from build123d import *

# Parameters (mm, degrees)
BOSS_EXTRUDE1_DEPTH = 30.48
BOSS_EXTRUDE2_DEPTH = 3.175
SKETCH3_W           = 3.436
SKETCH3_H           = 3.81
CUT_EXTRUDE1_DEPTH  = 12.7
SKETCH5_R           = 2.45
CUT_EXTRUDE2_DEPTH  = 1.5875
SKETCH6_W           = 23
SKETCH6_H           = 27.305
SKETCH6_R           = 4.5
BOSS_EXTRUDE3_DEPTH = 3.2
FILLET3_R           = 0.5
FILLET1_R           = 0.5
FILLET5_R           = 0.5
FILLET4_R           = 0.5
FILLET6_R           = 0.5


with BuildPart() as part:
    # Sketch1 → Boss-Extrude1 (new body)
    with BuildSketch(Plane(origin=(0, 0, 0), x_dir=(1, 0, 0), z_dir=(0, 1, 0))):
        Polygon((4.5, -6.1), (4.5, -7.6875), (13.088, -7.6875), (13.088, 7.6875), (-13.088, 7.6875), (-13.088, -7.6875), (-4.5, -7.6875), (-4.5, -6.1), (-11.5, -6.1), (-11.5, 6.1), (11.5, 6.1), (11.5, -6.1), align=None)
    extrude(amount=BOSS_EXTRUDE1_DEPTH)

    # Sketch2 → Boss-Extrude2 (add)
    with BuildSketch(Plane.XZ):
        Polygon((11.5, 0), (11.5, 6.1), (9.5, 6.1), (9.5, 0), (-1.5, 0), (-1.5, 6.1), (-11.5, 6.1), (-11.5, -6.1), (11.5, -6.1), align=None)
    extrude(amount=-BOSS_EXTRUDE2_DEPTH)

    # Sketch3 → Cut-Extrude1 (cut)
    with BuildSketch(Plane(origin=(0, 30.48, 0), x_dir=(1, 0, 0), z_dir=(0, 1, 0))):
        with Locations((-11.37, -2.925)):
            Rectangle(SKETCH3_W, SKETCH3_H)
    cut_extrude1 = extrude(amount=-CUT_EXTRUDE1_DEPTH, mode=Mode.SUBTRACT)

    # Mirror1: Cut-Extrude1 across plane
    add(cut_extrude1.mirror(Plane(origin=(0, 0, 0), x_dir=(0, 0, 1), z_dir=(1, 0, 0))), mode=Mode.SUBTRACT)

    # Sketch5 → Cut-Extrude2 (cut)
    with BuildSketch(Plane(origin=(0, 0, -7.6875), x_dir=(-1, 0, 0), z_dir=(0, 0, -1))):
        with Locations((0, 8.466666667)):
            Circle(SKETCH5_R)
        with Locations((0, 22.013333333)):
            Circle(SKETCH5_R)
    extrude(amount=-CUT_EXTRUDE2_DEPTH, mode=Mode.SUBTRACT)

    # Sketch6 → Boss-Extrude3 (add)
    with BuildSketch(Plane.XY.offset(-6.1)):
        with Locations((0, 16.8275)):
            Rectangle(SKETCH6_W, SKETCH6_H)
        with Locations((0, 22.013333333)):
            Circle(SKETCH6_R, mode=Mode.SUBTRACT)
        with Locations((0, 8.466666667)):
            Circle(SKETCH6_R, mode=Mode.SUBTRACT)
    extrude(amount=BOSS_EXTRUDE3_DEPTH)

    # Fillet3
    fillet3_edges = [part.edges().sort_by_distance(p)[0] for p in [
        (11.5, 3.175, 1.6),
        (0, 3.175, -2.9),
        (11.5, 16.8275, -2.9),
        (11.5, 16.8275, 6.1),
    ]]
    fillet(fillet3_edges, radius=FILLET3_R)

    # Fillet1
    fillet1_edges = [part.edges().sort_by_distance(p)[0] for p in [
        (-11.5, 17.0775, -2.9),
        (-11.5, 3.321446609, -2.753553391),
        (4.5, 15.24, 6.1),
        (-11.5, 3.175, 1.85),
        (-8, 3.175, 6.1),
    ]]
    fillet(fillet1_edges, radius=FILLET1_R)

    # Fillet5
    # the kernel refuses this fillet: 0.5 mm, written as the material it adds along each edge
    with BuildSketch(Plane(origin=(-13.088, 17.78, 4.83), x_dir=(0, 1, 0), z_dir=(1, 0, 0)), Plane(origin=(11.5, 17.78, 1.02), x_dir=(0, 0, 1), z_dir=(1, 0, 0))) as fillet5_piece_1:
        with BuildLine():
            CenterArc((FILLET5_R, -FILLET5_R), FILLET5_R, 90, 90)
            Line((0, -FILLET5_R), (0, 0))
            Line((0, 0), (FILLET5_R, 0))
        make_face()
    extrude(amount=1.588)
    with BuildSketch(Plane(origin=(-11.5, 17.78, 1.02), x_dir=(0, 0, 1), z_dir=(-1, 0, 0)), Plane(origin=(13.088, 17.78, 4.83), x_dir=(0, 1, 0), z_dir=(-1, 0, 0))) as fillet5_piece_2:
        with BuildLine():
            CenterArc((FILLET5_R, FILLET5_R), FILLET5_R, 180, 90)
            Line((0, FILLET5_R), (0, 0))
            Line((0, 0), (FILLET5_R, 0))
        make_face()
    extrude(amount=1.588)
    # the kernel refuses this fillet: 0.5 mm, written as the material it takes off along each edge
    with BuildSketch(Plane(origin=(-4.5, 3.675, 6.1), x_dir=(0, 0, 1), z_dir=(0, 1, 0))) as fillet5_2_piece_1:
        with BuildLine():
            CenterArc((FILLET5_R, -FILLET5_R), FILLET5_R, 90, 90)
            Line((0, -FILLET5_R), (0, 0))
            Line((0, 0), (FILLET5_R, 0))
        make_face()
    extrude(amount=28.055, mode=Mode.SUBTRACT)
    with BuildSketch(Plane(origin=(-4.5, 3.675, 5.6), x_dir=(0, 0.8017442392976493, -0.5976672776328263), z_dir=(0, 0.5976672776328263, 0.8017442392976493))) as fillet5_2_piece_2_section:
        with BuildLine():
            CenterArc((0.5 + FILLET5_R, FILLET5_R), FILLET5_R, 180, 90)
            Line((0.5, FILLET5_R), (0.5, 0))
            Line((0.5, 0), (0.5 + FILLET5_R, 0))
        make_face()
    fillet5_2_piece_2 = revolve(axis=Axis((-4.5, 3.675, 5.6), (-1, 0, 0)), revolution_arc=233.296989237, mode=Mode.PRIVATE)
    fillet5_2_piece_2 = split(fillet5_2_piece_2, bisect_by=Plane(origin=(-4.655814155, 3.175, 5.974969475), z_dir=(0, 1, 0)), keep=Keep.TOP, mode=Mode.PRIVATE)
    add(fillet5_2_piece_2, mode=Mode.SUBTRACT)
    with BuildSketch(Plane(origin=(-4.5, 3.675, 5.6), x_dir=(0, 0.8017442392976493, -0.5976672776328263), z_dir=(0, 0.5976672776328263, 0.8017442392976493))) as fillet5_2_piece_3_section:
        with BuildLine():
            CenterArc((0.5 + FILLET5_R, FILLET5_R), FILLET5_R, 180, 90)
            Line((0.5, FILLET5_R), (0.5, 0))
            Line((0.5, 0), (0.5 + FILLET5_R, 0))
        make_face()
    fillet5_2_piece_3 = revolve(axis=Axis((-4.5, 3.675, 5.6), (-1, 0, 0)), revolution_arc=233.296989237, mode=Mode.PRIVATE)
    fillet5_2_piece_3 = split(fillet5_2_piece_3, bisect_by=Plane(origin=(-4.518548164, 3.09595455, 6.1), z_dir=(0, 0, 1)), keep=Keep.TOP, mode=Mode.PRIVATE)
    add(fillet5_2_piece_3, mode=Mode.SUBTRACT)

    # Fillet4
    # the kernel refuses this fillet: 0.5 mm, written as the material it adds along each edge
    with BuildSketch(Plane(origin=(-11, 3.675, 5.6), x_dir=(-1, 0, 0), z_dir=(0, 0, 1))) as fillet4_piece_1_section:
        Polygon((0, 0), (FILLET4_R, 0), (FILLET4_R, FILLET4_R), (0, FILLET4_R), align=None)
    fillet4_piece_1 = extrude(amount=FILLET4_R, mode=Mode.PRIVATE)
    fillet4_piece_1 = fillet4_piece_1 - Plane(origin=(-11, 3.675, 5.6), x_dir=(0.7071067811865475, 0.7071067811865475, 0), z_dir=(0, 0, 1)) * Sphere(FILLET4_R, mode=Mode.PRIVATE)
    add(fillet4_piece_1)
    with BuildSketch(Plane(origin=(-11.5, 3.675, 6.1), x_dir=(1, 0, 0), z_dir=(0, 1, 0))) as fillet4_piece_2:
        with BuildLine():
            CenterArc((FILLET4_R, FILLET4_R), FILLET4_R, 180, 90)
            Line((0, FILLET4_R), (0, 0))
            Line((0, 0), (FILLET4_R, 0))
        make_face()
    extrude(amount=26.805)

    # Fillet6
    # the kernel refuses this fillet: 0.5 mm, written as the material it adds along each edge
    with BuildSketch(Plane(origin=(11, 3.675, 5.6), x_dir=(0, 0, 1), z_dir=(0, -1, 0))) as fillet6_piece_1_section:
        Polygon((0, 0), (FILLET6_R, 0), (FILLET6_R, -FILLET6_R), (0, -FILLET6_R), align=None)
    fillet6_piece_1 = extrude(amount=FILLET6_R, mode=Mode.PRIVATE)
    fillet6_piece_1 = fillet6_piece_1 - Plane(origin=(11, 3.675, 5.6), x_dir=(-0.7071067811865475, 0, -0.7071067811865475), z_dir=(0, -1, 0)) * Sphere(FILLET6_R, mode=Mode.PRIVATE)
    add(fillet6_piece_1)
    with BuildSketch(Plane(origin=(11, 3.175, 6.1), x_dir=(0, 0, -1), z_dir=(-1, 0, 0))) as fillet6_piece_2:
        with BuildLine():
            CenterArc((FILLET6_R, -FILLET6_R), FILLET6_R, 90, 90)
            Line((0, -FILLET6_R), (0, 0))
            Line((0, 0), (FILLET6_R, 0))
        make_face()
    extrude(amount=1.5)
    with BuildSketch(Plane(origin=(-1.5, 0, 0), x_dir=(1, 0, 0), z_dir=(0, 1, 0)), Plane(origin=(9.5, 0, 0), x_dir=(0, 0, 1), z_dir=(0, 1, 0)), Plane(origin=(9.5, 0, 6.1), x_dir=(-1, 0, 0), z_dir=(0, 1, 0))) as fillet6_piece_3:
        with BuildLine():
            CenterArc((FILLET6_R, -FILLET6_R), FILLET6_R, 90, 90)
            Line((0, -FILLET6_R), (0, 0))
            Line((0, 0), (FILLET6_R, 0))
        make_face()
    extrude(amount=3.175)
    with BuildSketch(Plane(origin=(11, 3.175, 6.1), x_dir=(0, 0, -1), z_dir=(-1, 0, 0))) as fillet6_piece_4a_section:
        with BuildLine():
            CenterArc((FILLET6_R, -FILLET6_R), FILLET6_R, 90, 90)
            Line((0, -FILLET6_R), (0, 0))
            Line((0, 0), (FILLET6_R, 0))
        make_face()
    fillet6_piece_4a = extrude(amount=2.75, mode=Mode.PRIVATE)
    fillet6_piece_4a = split(fillet6_piece_4a, bisect_by=Plane(origin=(9.5, 3.288197557, 5.986802443), z_dir=(-1, 0, 0)), keep=Keep.TOP, mode=Mode.PRIVATE)
    with BuildSketch(Plane(origin=(9.5, 0, 6.1), x_dir=(-1, 0, 0), z_dir=(0, 1, 0))) as fillet6_piece_4b_section:
        with BuildLine():
            CenterArc((FILLET6_R, -FILLET6_R), FILLET6_R, 90, 90)
            Line((0, -FILLET6_R), (0, 0))
            Line((0, 0), (FILLET6_R, 0))
        make_face()
    fillet6_piece_4b = extrude(amount=4.425, mode=Mode.PRIVATE)
    fillet6_piece_4b = split(fillet6_piece_4b, bisect_by=Plane(origin=(9.386802443, 3.175, 5.986802443), z_dir=(0, 1, 0)), keep=Keep.TOP, mode=Mode.PRIVATE)
    fillet6_piece_4 = fillet6_piece_4a & fillet6_piece_4b
    add(fillet6_piece_4)


solid = part.part
Geometry: final body of the model. Coordinates: model frame, mm. A direction names the side the tool comes from. Coordinates: 2 decimals unless noted, no trailing zeros. Order: outer loops, then holes, each group sorted by start corner. A loop starts at its lowest first (then second) coordinate and runs counter-clockwise, first axis right, second up.
1) First-contact query: P1, Ø0.8, axis at x = -12.5, z = 3, coming from the +Y side; P2, Ø5.5, axis at x = 0, y = 8.47, coming from the +Z side. Flat tips, straight axial feed; report the tip coordinate or a pass-through.
Result sheet:
P1: stops at y = 17.78
P2: stops at z = -6.1
2) Section C-C (z = -1.5). Return loops of the section in (x, y) (3 decimals).
Result sheet:
outline: (-13.088, 0) - (13.088, 0) - (13.088, 30.48) - (11.5, 30.48) - (11.5, 3.675) arc R0.5 cw to (11, 3.175) - (-11, 3.175) arc R0.5 cw to (-11.5, 3.675) - (-11.5, 30.48) - (-13.088, 30.48) - close
3) Ray query, probe 1 along Y at (x, z) = (0, -3.95); probe 2 along Z at (x, y) = (7.5, 4); probe 3 along X at (y, z) = (17, -2.25). Return the intervals inside material, ascending.
Result sheet:
probe 1: y = 0 to 3.97, 12.97 to 17.51, 26.51 to 30.48
probe 2: z = -7.69 to -2.9, 6.1 to 7.69
probe 3: x = -13.09 to -11.5, 11.5 to 13.09
4) Section A-A (x = 0). Give the number of separate pieces and of enclosed holes in the cut face, then the cut area to 3 significant figures.
Result sheet:
separate pieces: 3
enclosed holes: 0
area: 82.0 mm2
5) Section B-B (y = 28.5). Return loops of the section in (x, z).
Result sheet:
outline: (-13.09, -7.69) - (13.09, -7.69) - (13.09, 1.02) - (11.5, 1.02) - (11.5, -2.4) arc R0.5 cw to (11, -2.9) - (-11, -2.9) arc R0.5 cw to (-11.5, -2.4) - (-11.5, 1.02) - (-13.09, 1.02) - close; (-13.09, 4.83) - (-11.5, 4.83) - (-11.5, 5.6) arc R0.5 cw to (-11, 6.1) - (-5, 6.1) arc R0.5 ccw to (-4.5, 6.6) - (-4.5, 7.69) - (-13.09, 7.69) - close; (4.5, 6.6) arc R0.5 ccw to (5, 6.1) - (11, 6.1) arc R0.5 cw to (11.5, 5.6) - (11.5, 4.83) - (13.09, 4.83) - (13.09, 7.69) - (4.5, 7.69) - close
6) Draft query along Z for faces 1 (the flat face through (2, 24, -6.1)), 2 (the flat face through (-8, 17, 6.1)), 3 (the flat face through (-13.088, 15, 0)). Return one class per face: released by +Z, released by -Z, zero draft, split by the parting line, or undercut.
Result sheet:
face 1: released by +Z
face 2: undercut
face 3: zero draft
7) Section D-D (x = 5.5). Return loops of the section in (y, z) (1 decimal).
Result sheet:
outline: (0, -7.7) - (30.5, -7.7) - (30.5, -2.9) - (3.7, -2.9) arc R0.5 cw to (3.2, -2.4) - (3.2, 0) - (0, 0) - close; (0, 6.1) - (30.5, 6.1) - (30.5, 7.7) - (0, 7.7) - close
8) Set-up query: faces 4 (the flat face through (13.088, 15, 0)), 5 (the cylindrical face through (2.419, 25.808, -4.522)), 6 (the flat face through (4.5, 15, 7)), 7 (the flat face through (-11.5, 14, 2)), 8 (the flat face through (12, 24, 1.02)). Return all of +Z, -Z, +X, -X, +Y, -Y with unobstructed straight access to the full face (end or side cutting, diameter ignored); none if empty.
Result sheet:
face 4: +Z, -Z, +X, +Y, -Y
face 5: +Z
face 6: +Z, +Y, -Y
face 7: +Y
face 8: +X, -X, +Y
